```python
from build123d import *

# Parameters (mm, degrees)
F0_R     = 55.3
F1_DEPTH = 15
F2_R     = 53.9
F3_DEPTH = 5
F4_R     = 15
F5_DEPTH = 25
F7_DEPTH = 25
F8_R     = 0.5
F9_R     = 0.2


with BuildPart() as f1:
    # F0 (on Front) → F1 (new body)
    with BuildSketch(Plane.XZ):
        Circle(F0_R)
    extrude(amount=F1_DEPTH)

    # F2 (on face) → F3 (join)
    with BuildSketch(Plane.XZ.offset(15)):
        Circle(F2_R)
    extrude(amount=F3_DEPTH)

    # F4 (on face) → F5 (cut)
    with BuildSketch(Plane.XZ.offset(20)):
        Circle(F4_R)
    extrude(amount=-F5_DEPTH, mode=Mode.SUBTRACT)

    # F6 (on face) → F7 (cut)
    with BuildSketch(Plane(origin=(0, 0, 0), x_dir=(-1, 0, 0), z_dir=(0, 1, 0))):
        with BuildLine():
            Line((37.5, 40.6428345468), (37.5, -40.6428345468))
            ThreePointArc((37.5, -40.6428345468), (50.6549109169, -22.1849047778), (55.3, 0))
            ThreePointArc((55.3, 0), (50.6549109169, 22.1849047778), (37.5, 40.6428345468))
        make_face()
        with BuildLine():
            ThreePointArc((-37.5, 40.6428345468), (-55.3, 0), (-37.5, -40.6428345468))
            Line((-37.5, -40.6428345468), (-37.5, 40.6428345468))
        make_face()
    extrude(amount=-F7_DEPTH, mode=Mode.SUBTRACT)

    # F8
    f8_edges = [f1.edges().sort_by_distance(p)[0] for p in [
        (37.5, 0, 0),
        (0, 0, 55.3),
        (0, 0, -55.3),
        (-37.5, 0, 0),
    ]]
    fillet(f8_edges, radius=F8_R)

    # F9
    f9_edges = [f1.edges().sort_by_distance(p)[0] for p in [
        (0, -20, -53.9),
        (0, -20, 53.9),
        (0, -15, 55.3),
        (0, -15, -55.3),
    ]]
    fillet(f9_edges, radius=F9_R)


solid = f1.part
```
Geometry: final body of the model. Coordinates: model frame, mm. A direction names the side the tool comes from. Give positions to 0.01 mm unless a question says otherwise; leave off trailing zeros. Write each loop counter-clockwise with the first axis right and the second up, starting at its lowest first coordinate (ties: lowest second). Pieces come first, ordered by that corner, then holes.
1. Pin query (flat end, axial travel): P1, Ø8, axis at x = -16, y = -15, coming from the -Z side; P2, Ø12, axis at x = -11, y = -9.5, coming from the +Z side. Return the tip coordinate at first contact, or that it passes through.
2. Line query: probe 1 along Z at (x, y) = (0, -15.5); probe 2 along Z at (x, y) = (0.5, -10); probe 3 along X at (y, z) = (-6.5, 13.5). Output: solid intervals per line, ascending.
3. Draft query along Z for faces 1 (the cylindrical face through (-14.985, -10.14, 0.66)), 2 (the cylindrical face through (0.581, -17.366, 53.897)), 3 (the flat face through (-0.2, -15, 54.2)). Return one class per face: released by +Z, released by -Z, zero draft, split by the parting line, or undercut.
4. Section query A-A, the plane z = 0. Return loops of the section in (x, y), then the cut area to 3 significant figures.
5. Section query B-B, the plane x = 0. Return loops of the section in (y, z), then the cut area to 3 significant figures.
6. Section query D-D, the plane y = -8. Return loops of the section in (x, z), then the cut area to 3 significant figures.
7. Section query C-C, the plane y = -18. Return loops of the section in (x, z), then the cut area to 3 significant figures.
8. Reachability of faces 4 (the flat face through (-37.5, -10, 1)), 5 (the flat face through (-0.2, -15, -54.2)) from +Z, -Z, +X, -X, +Y, -Y: full face, straight path, thin tool, end or side. Return the list, or none.
Computed:
1. P1: stops at z = -53.98
1. P2: stops at z = 55.07
2. probe 1: z = -53.9 to -15, 15 to 53.9
2. probe 2: z = -55.3 to -14.99, 14.99 to 55.3
2. probe 3: x = -37.5 to -6.54, 6.54 to 37.5
3. face 1: undercut
3. face 2: released by +Z
3. face 3: zero draft
4. outline: (-37.5, -20) - (-15, -20) - (-15, 0) - (-37, 0) arc R0.5 ccw to (-37.5, -0.5) - close; (15, -20) - (37.5, -20) - (37.5, -0.5) arc R0.5 ccw to (37, 0) - (15, 0) - close
4. area: 900 mm2
5. outline: (-20, -53.7) arc R0.2 ccw to (-19.8, -53.9) - (-15, -53.9) - (-15, -55.1) arc R0.2 ccw to (-14.8, -55.3) - (-0.5, -55.3) arc R0.5 ccw to (0, -54.8) - (0, -15) - (-20, -15) - close; (-20, 15) - (0, 15) - (0, 54.8) arc R0.5 ccw to (-0.5, 55.3) - (-14.8, 55.3) arc R0.2 ccw to (-15, 55.1) - (-15, 53.9) - (-19.8, 53.9) arc R0.2 ccw to (-20, 53.7) - close
5. area: 1,600 mm2
6. outline: (-37.5, -40.64) arc R55.3 ccw to (37.5, -40.64) - (37.5, 40.64) arc R55.3 ccw to (-37.5, 40.64) - close; hole circle Ø30 at (0, 0)
6. area: 6,900 mm2
7. outline: (-37.5, -38.72) arc R53.9 ccw to (37.5, -38.72) - (37.5, 38.72) arc R53.9 ccw to (-37.5, 38.72) - close; hole circle Ø30 at (0, 0)
7. area: 6,670 mm2
8. face 4: +Z, -Z, -X, +Y, -Y
8. face 5: -Z, -Y
